The listing builds one solid part. Answer for the finished solid, in the listing's coordinates (mm). A direction names the side the tool comes from. Coordinates: 2 decimals unless noted, no trailing zeros. Loops run counter-clockwise (first coordinate to the right, second up) from the corner with the lowest first, then second, coordinate; pieces in that order, holes last. Notation, with made-up numbers: (50.5, 27.25) - (90.5, 27.25) arc R24 cw to (90.5, 55.25) - close; hole circle Ø3 at (16.25, 34). An arc over 180 degrees is marked (long way). One line per question, with ' | ' between items.
from build123d import *

# Parameters (mm, degrees)
F0_R     = 65
F1_DEPTH = 10
F2_R     = 2
F3_DEPTH = 8


with BuildPart() as f1:
    # F0 (on Top) → F1 (new body)
    with BuildSketch(Plane.XY):
        Circle(F0_R)
    extrude(amount=F1_DEPTH)

    # F2 (on face) → F3 (cut)
    with BuildSketch(Plane(origin=(0, 0, 0), x_dir=(1, 0, 0), z_dir=(0, 0, -1))):
        with Locations((0, 50)):
            Circle(F2_R)
        with Locations((50, 0)):
            Circle(F2_R)
        with Locations((0, -50)):
            Circle(F2_R)
        with Locations((-50, 0)):
            Circle(F2_R)
    extrude(amount=-F3_DEPTH, mode=Mode.SUBTRACT)


solid = f1.part
Item 1: Which of the six approach directions +Z, -Z, +X, -X, +Y, -Y give full straight-line access (tool end or side, diameter ignored) to faces 4 (the face through (-1, 1, 0)), 5 (the face through (0, 50, 8))?
Taken from the geometry:
face 4: -Z, +X, -X, +Y, -Y | face 5: -Z
Item 2: Find section A-A, the plane y = 0. Write down the section's boundary in (x, z), plus the area to 3 significant figures.
Taken from the geometry:
outline: (-65, 0) - (-52, 0) - (-52, 8) - (-48, 8) - (-48, 0) - (48, 0) - (48, 8) - (52, 8) - (52, 0) - (65, 0) - (65, 10) - (-65, 10) - close | area: 1,240 mm2
Item 3: Each of these flat-tipped pins is pushed along its axis until it touches: pin 1 Ø1.5 at (x, z) = (-7, 1.5) entering from +Y; pin 2 Ø4 at (x, z) = (-16, 2.5) entering from -Y; pin 3 Ø2.5 at (x, y) = (0, 50) entering from -Z. Where does it stop, or does it pass through?
Taken from the geometry:
pin 1: stops at y = 64.7 | pin 2: stops at y = -63.47 | pin 3: stops at z = 8
Item 4: Find section C-C, the plane x = 16. Write down the section's boundary in (y, z).
Taken from the geometry:
outline: (-63, 0) - (63, 0) - (63, 10) - (-63, 10) - close
Item 5: Find the intervals of material crossed by line 1 (Y direction, x = -50, z = 6.25); line 2 (X direction, y = -50.5, z = 7.5), in increasing order. Write a range as [from, to].
Taken from the geometry:
line 1: y = [-41.53, -2], [2, 41.53] | line 2: x = [-40.92, -1.94], [1.94, 40.92]
Item 6: The mould has two halves that part along Y. Classify faces 1 (the face through (-1, 1, 10)), 2 (the face through (0.923, -48.226, 3.944)), 3 (the face through (62, 19.52, 4.93)): pulls with the +Y half, pulls with the -Y half, needs draft (parallel to the pull), parting line crosses it, or undercut.
Taken from the geometry:
face 1: needs draft | face 2: undercut | face 3: parting line crosses it
Item 7: Find section B-B, the plane x = 50. Write down the section's boundary in (y, z), plus the area to 3 significant figures.
Taken from the geometry:
outline: (-41.53, 0) - (-2, 0) - (-2, 8) - (2, 8) - (2, 0) - (41.53, 0) - (41.53, 10) - (-41.53, 10) - close | area: 799 mm2
